The model under review builds one solid part; all positions refer to its coordinate system, in mm. Face numbers are marked on the shaded views. Coordinates: 2 decimals unless noted, no trailing zeros. Loops run counter-clockwise (first coordinate to the right, second up) from the corner with the lowest first, then second, coordinate; pieces in that order, holes last. Notation, with made-up numbers: (42.25, -10) - (47.25, -10) arc R20 ccw to (47.25, 0) - close; hole circle Ø10 at (24, 46.25). An arc over 180 degrees is marked (long way). Use a Markdown table: item, result. Add a question column.
1) To check wall thickness, follow L1, parallel to X at y = -23.5, z = 62; L2, parallel to Z at x = 1, y = -54.5; L3, parallel to Z at x = -29.5, y = -11. State the ranges of each line that lie inside material, in increasing order. Write a range as [from, to].
2) The part is to be moulded in two halves that separate along X. For the marked faces 1, 2 and 3, say which applies: pulls with the +X half, pulls with the -X half, needs draft (parallel to the pull), parting line crosses it, or undercut.
3) Add section C-C, the plane y = -48. Give the boundary of the cut face in (x, z).
4) Add section D-D, the plane x = 30. Give the number of separate pieces and of enclosed holes in the cut face, and give its area (3 significant figures).
5) Add section B-B, the plane z = -3.5. Give the boundary of the cut face in (x, y).
6) Add section A-A, the plane x = 0. Give the boundary of the cut face in (y, z), and give its area (3 significant figures).
7) Clearance check with flat-ended pins moving along their axes: pin 1 (2 mm diameter, centred on x = -28, y = -92, fed in from -Z); pin 2 (4 mm diameter, centred on y = -77, z = -42.5, fed in from +X); pin 3 (3 mm diameter, centred on x = 24, z = -67.5, fed in from -Y). State where each tip first meets the part, or that it passes through.
```python
from build123d import *

# Parameters (mm, degrees)
F0_R         = 20.9202002185
F1_DEPTH     = 104.14
F2_T1_DEPTH  = 101.6
F2_T3_DEPTH  = 76.2
F2_T5_DEPTH  = 50.8
F2_T8_ANGLE  = 90
F2_T10_ANGLE = 90
F2_T12_ANGLE = 90
F2_T14_ANGLE = 90
F3_R         = 12.7
F4_R         = 38.1
F5_DEPTH     = 104.1410001


# Not quite as in the source:
# - a fillet or chamfer that OpenCascade refuses, or shapes differently, is made with other operations: its cross-section is extruded or revolved along the edge and cut away or added


with BuildPart() as f1:
    # F0 (on Front) → F1 (new body)
    with BuildSketch(Plane.XZ):
        with BuildLine():
            Line((0, 101.6), (-50.8, 101.6))
            ThreePointArc((-50.8, 101.6), (-86.7210244843, 86.7210244843), (-101.6, 50.8))
            Line((-101.6, 50.8), (-101.6, -25.4))
            ThreePointArc((-101.6, -25.4), (-79.2815367264, -79.2815367264), (-25.4, -101.6))
            Line((-25.4, -101.6), (0, -101.6))
            Line((0, -101.6), (0, 101.6))
        make_face()
        with Locations((-37.8764681518, 59.70396474)):
            Circle(F0_R, mode=Mode.SUBTRACT)
        with BuildLine():
            Line((50.8, 101.6), (0, 101.6))
            Line((0, 101.6), (0, -101.6))
            Line((0, -101.6), (25.4, -101.6))
            ThreePointArc((25.4, -101.6), (79.2815367264, -79.2815367264), (101.6, -25.4))
            Line((101.6, -25.4), (101.6, 50.8))
            ThreePointArc((101.6, 50.8), (86.7210244843, 86.7210244843), (50.8, 101.6))
        make_face()
        with Locations((37.8764681518, 59.70396474)):
            Circle(F0_R, mode=Mode.SUBTRACT)
    extrude(amount=F1_DEPTH)

    # F2: fillet of radius 50.8 on 1 edges, made by hand

    # F2_s2 → F2_t1 (cut)
    with BuildSketch(Plane.YZ.offset(-50.8)):
        with BuildLine():
            ThreePointArc((-53.34, 101.6), (-89.2610244843, 86.7210244843), (-104.14, 50.8))
            Line((-104.14, 50.8), (-104.14, 101.6))
            Line((-104.14, 101.6), (-53.34, 101.6))
        make_face()
    extrude(amount=F2_T1_DEPTH, mode=Mode.SUBTRACT)

    # F2_s4 → F2_t3 (cut)
    with BuildSketch(Plane.XY.offset(-25.4)):
        with BuildLine():
            ThreePointArc((-101.6, -53.34), (-86.7210244843, -89.2610244843), (-50.8, -104.14))
            Line((-50.8, -104.14), (-101.6, -104.14))
            Line((-101.6, -104.14), (-101.6, -53.34))
        make_face()
        with BuildLine():
            ThreePointArc((101.6, -53.34), (86.7210244843, -89.2610244843), (50.8, -104.14))
            Line((50.8, -104.14), (101.6, -104.14))
            Line((101.6, -104.14), (101.6, -53.34))
        make_face()
    extrude(amount=F2_T3_DEPTH, mode=Mode.SUBTRACT)

    # F2_s6 → F2_t5 (cut)
    with BuildSketch(Plane.YZ.offset(-25.4)):
        with BuildLine():
            ThreePointArc((-53.34, -101.6), (-89.2610244843, -86.7210244843), (-104.14, -50.8))
            Line((-104.14, -50.8), (-104.14, -101.6))
            Line((-104.14, -101.6), (-53.34, -101.6))
        make_face()
    extrude(amount=F2_T5_DEPTH, mode=Mode.SUBTRACT)

    # F2_s7 → F2_t8 (revolve, cut)
    with BuildSketch(Plane.YZ.offset(-50.8)):
        with BuildLine():
            ThreePointArc((-53.34, 101.6), (-89.2610244843, 86.7210244843), (-104.14, 50.8))
            Line((-104.14, 50.8), (-104.14, 101.6))
            Line((-104.14, 101.6), (-53.34, 101.6))
        make_face()
    revolve(axis=Axis((-50.8, -104.14, 50.8), (0, -1, 0)), revolution_arc=F2_T8_ANGLE, mode=Mode.SUBTRACT)

    # F2_s9 → F2_t10 (revolve, cut)
    with BuildSketch(Plane.XY.offset(-25.4)):
        with BuildLine():
            ThreePointArc((-101.6, -53.34), (-86.7210244843, -89.2610244843), (-50.8, -104.14))
            Line((-50.8, -104.14), (-101.6, -104.14))
            Line((-101.6, -104.14), (-101.6, -53.34))
        make_face()
    revolve(axis=Axis((-25.4, -104.14, -25.4), (0, -1, 0)), revolution_arc=F2_T10_ANGLE, mode=Mode.SUBTRACT)

    # F2_s11 → F2_t12 (revolve, cut)
    with BuildSketch(Plane.YZ.offset(25.4)):
        with BuildLine():
            ThreePointArc((-53.34, -101.6), (-89.2610244843, -86.7210244843), (-104.14, -50.8))
            Line((-104.14, -50.8), (-104.14, -101.6))
            Line((-104.14, -101.6), (-53.34, -101.6))
        make_face()
    revolve(axis=Axis((25.4, -104.14, -25.4), (0, -1, 0)), revolution_arc=F2_T12_ANGLE, mode=Mode.SUBTRACT)

    # F2_s13 → F2_t14 (revolve, cut)
    with BuildSketch(Plane.XY.offset(50.8)):
        with BuildLine():
            ThreePointArc((101.6, -53.34), (86.7210244843, -89.2610244843), (50.8, -104.14))
            Line((50.8, -104.14), (101.6, -104.14))
            Line((101.6, -104.14), (101.6, -53.34))
        make_face()
    revolve(axis=Axis((50.8, -104.14, 50.8), (0, -1, 0)), revolution_arc=F2_T14_ANGLE, mode=Mode.SUBTRACT)

    # F3
    f3_edges = [f1.edges().sort_by_distance(p)[0] for p in [
        (-86.721024, 0, 86.721024),
    ]]
    fillet(f3_edges, radius=F3_R)

    # F4 (on face) → F5 (cut, through all)
    with BuildSketch(Plane.XZ.offset(104.14)):
        with Locations((0, -31.9225803405)):
            Circle(F4_R)
    extrude(amount=-F5_DEPTH, mode=Mode.SUBTRACT)


solid = f1.part
```
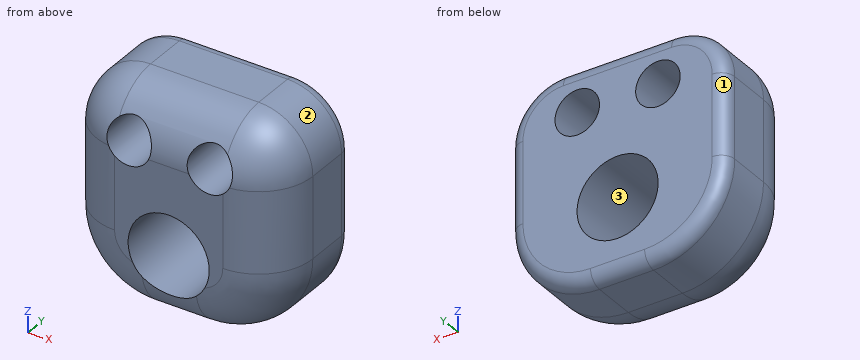
From the geometry:
| question | item | result |
|---|---|---|
| 1 | L1 | x = [-100.35, -58.67], [-17.08, 17.08], [58.67, 100.35] |
| 1 | L2 | z = [-101.59, -70.01], [6.16, 101.59] |
| 1 | L3 | z = [-101.38, -56.03], [-7.81, 40.53], [78.87, 101.49] |
| 2 | face 1 | pulls with the -X half |
| 2 | face 2 | pulls with the +X half |
| 2 | face 3 | undercut |
| 3 | outline | (-101.6, -25.4) arc R76.2 ccw to (-25.4, -101.6) - (25.4, -101.6) arc R76.2 ccw to (101.6, -25.4) - (101.6, 50.8) arc R50.8 ccw to (50.8, 101.6) - (-50.8, 101.6) arc R50.8 ccw to (-101.6, 50.8) - close; hole circle Ø41.84 at (-37.88, 59.7); hole circle Ø76.2 at (0, -31.92); hole circle Ø41.84 at (37.88, 59.7) |
| 4 | separate pieces | 3 |
| 4 | enclosed holes | 0 |
| 4 | area | 11,100 mm^2 |
| 5 | outline | (-101.6, -53.34) arc R50.8 ccw to (-50.8, -104.14) - (-25.37, -104.14) - (-25.37, 0) - (-88.9, 0) arc R12.7 ccw to (-101.6, -12.7) - close; (25.37, -104.14) - (50.8, -104.14) arc R50.8 ccw to (101.6, -53.34) - (101.6, -12.7) arc R12.7 ccw to (88.9, 0) - (25.37, 0) - close |
| 6 | outline | (-104.14, 6.18) - (0, 6.18) - (0, 88.9) arc R12.7 ccw to (-12.7, 101.6) - (-53.34, 101.6) arc R50.8 ccw to (-104.14, 50.8) - close; (-100.36, -70.02) arc R50.8 ccw to (-53.34, -101.6) - (-12.7, -101.6) arc R12.7 ccw to (0, -88.9) - (0, -70.02) - close |
| 6 | area | 12,100 mm^2 |
| 7 | pin 1 | stops at z = -84.84 |
| 7 | pin 2 | stops at x = 94.78 |
| 7 | pin 3 | stops at y = -101.81 |
